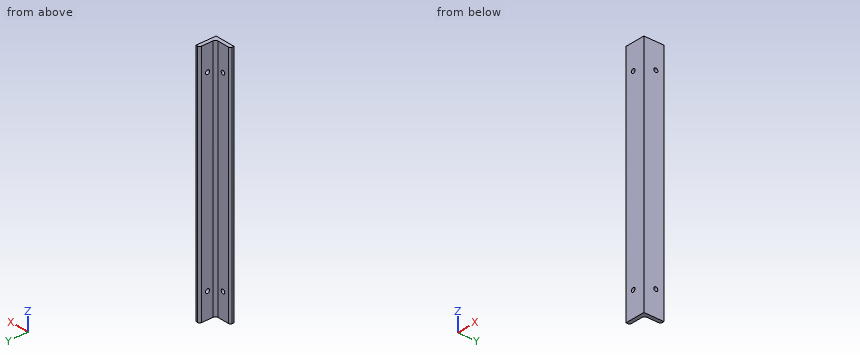
from build123d import *

# Parameters (mm, degrees)
BOSS_EXTRUDE1_DEPTH    = 152.4
F_10_CLEARANCE_HOLE2_D = 5.1054
F_10_CLEARANCE_HOLE3_D = 5.1054


with BuildPart() as part:
    # Sketch2 → Boss-Extrude1 (new, symmetric)
    with BuildSketch(Plane.XY):
        with BuildLine():
            Line((-12.7, 0), (12.7, 0))
            Line((12.7, 0), (12.7, 25.4))
            Line((12.7, 25.4), (10.31875, 25.4))
            ThreePointArc((10.31875, 25.4), (8.634951977, 24.702548023), (7.9375, 23.01875))
            Line((7.9375, 23.01875), (7.9375, 7.9375))
            ThreePointArc((7.9375, 7.9375), (7.00756403, 5.69243597), (4.7625, 4.7625))
            Line((4.7625, 4.7625), (-10.31875, 4.7625))
            ThreePointArc((-10.31875, 4.7625), (-12.002548023, 4.065048023), (-12.7, 2.38125))
            Line((-12.7, 2.38125), (-12.7, 0))
        make_face()
    extrude(amount=BOSS_EXTRUDE1_DEPTH, both=True)

    # #10 Clearance Hole2 (through all)
    with Locations(Plane(origin=(12.7, 0, 0), x_dir=(0, 0, -1), z_dir=(1, 0, 0))):
        with Locations((-120.65, 15.113), (120.65, 15.113)):
            Hole(F_10_CLEARANCE_HOLE2_D / 2)

    # #10 Clearance Hole3 (through all)
    with Locations(Plane(origin=(0, 0, 0), x_dir=(-1, 0, 0), z_dir=(0, -1, 0))):
        with Locations((2.413, -120.65), (2.413, 120.65)):
            Hole(F_10_CLEARANCE_HOLE3_D / 2)


solid = part.part
The model under review builds one solid part; all positions refer to its coordinate system, in mm. Round coordinates to 2 decimals unless told otherwise and drop trailing zeros. Answer as CSV lines item,"result". Start each with the question number.
Q1. Wall thickness on line 1 along Y through (x, z) = (10.45, 120.65); line 2 along Z through (x, y) = (-2.75, 2); line 3 along X through (y, z) = (2.8, 120.65): over which ranges is each line inside the solid? List them lowest first.
Q2. Clearance check with flat-ended pins moving along their axes: P1, Ø4, axis at y = 15.113, z = -120.65, coming from the +X side; P2, Ø12, axis at y = 8.5, z = 72, coming from the -X side; P3, Ø8, axis at x = -2.413, z = 120.65, coming from the +Y side; P4, Ø12, axis at y = 19, z = 43.5, coming from the -X side. State where each tip first meets the part, or that it passes through.
Q3. Consider section A-A, the plane z = 120.65. State how many separate pieces and enclosed holes the cut face has, then the cut area to 3 significant figures.
Result set:
1,line 1,"y = 0 to 12.56, 17.67 to 25.4"
1,line 2,"z = -152.4 to -123.18, -118.12 to 118.12, 123.18 to 152.4"
1,line 3,"x = -12.66 to -4.97, 0.14 to 12.7"
2,P1,"passes through"
2,P2,"stops at x = -12.7"
2,P3,"stops at y = 4.76"
2,P4,"stops at x = 7.94"
3,separate pieces,"3"
3,enclosed holes,"0"
3,area,"170 mm²"
